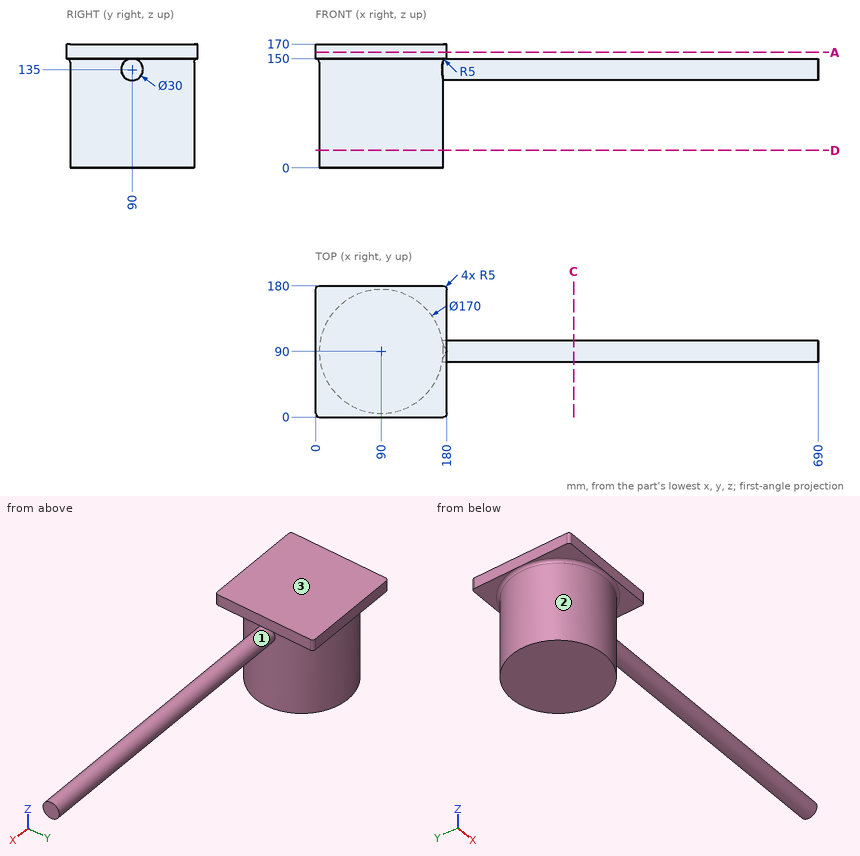
Part print with two shaded views. Sizes in mm from the minimum x, y, z corner. A direction names the side the tool comes from. Give positions to 0.01 mm unless a question says otherwise; leave off trailing zeros. Order: outer loops, then holes, each group sorted by start corner. A loop starts at its lowest first (then second) coordinate and runs counter-clockwise, first axis right, second up. Notation, with made-up numbers: M -0.5,81 L 11.5,81 A24 cw 11.5,113 Z; hole C 45,45 d7. An arc over 180 degrees is marked long. Put each result on its own line as item: value.
Item 1: Cut at D-D on z = 24. Write the cut outline in (x, y).
Results are:
outline: C 90,90 d170
Item 2: Cut at C-C on x = 354. Write the cut outline in (y, z).
Results are:
outline: C 90,135 d30
Item 3: Drop flat-ended pins along their axis: pin 1 Ø3 at (y, z) = (144, 116.5) entering from -X; pin 2 Ø1 at (x, z) = (163.5, 82.5) entering from +Y; pin 3 Ø22 at (y, z) = (116, 162) entering from +X. Give the stop position or say it passes through.
Results are:
pin 1: x = 23.15
pin 2: y = 133.54
pin 3: x = 180
Item 4: Cut at A-A on z = 158.5. Write the cut outline in (x, y).
Results are:
outline: M 0,5 A5 ccw 5,0 L 175,0 A5 ccw 180,5 L 180,175 A5 ccw 175,180 L 5,180 A5 ccw 0,175 Z
Item 5: Which spindle directions (+Z, -Z, +X, -X, +Y, -Y) get a long thin tool onto all of the face, cutting with end or side? Do the marked faces 1, 2 and 3. Say none if no direction does.
Results are:
face 1: +X
face 2: -Z
face 3: +Z, +X, -X, +Y, -Y
Item 6: Wall check: probe 1 along X at (y, z) = (110, 162.5); probe 2 along X at (y, z) = (87, 13); probe 3 along Y at (x, z) = (99, 9). Give the ranges that are in metal, low to high.
Results are:
probe 1: 0 to 180
probe 2: 5.05 to 174.95
probe 3: 5.48 to 174.52
